Can you work these out from the model? Positions are in its coordinate system, mm. Face numbers are marked on the shaded views. A direction names the side the tool comes from. Round coordinates to 2 decimals unless told otherwise and drop trailing zeros. Loops run counter-clockwise (first coordinate to the right, second up) from the corner with the lowest first, then second, coordinate; pieces in that order, holes last. Notation, with made-up numbers: (66, 11.25) -> (77, 11.25) arc R19 ccw to (77, 27.25) -> close; hole circle Ø1 at (-7.75, -39). An arc over 180 degrees is marked (long way). Use a Markdown table: item, result.
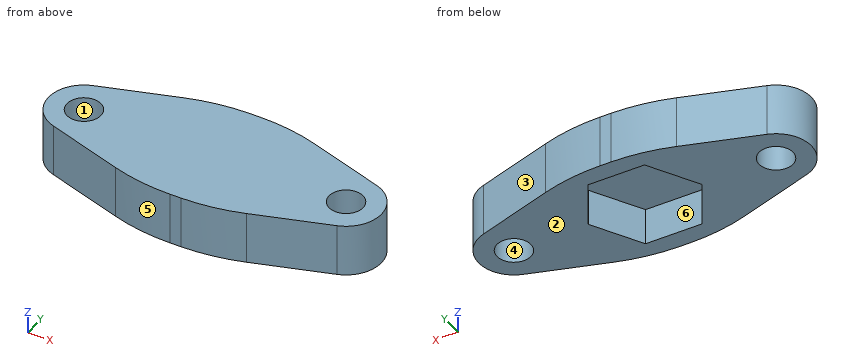
from build123d import *

# Parameters (mm, degrees)
SKETCH1_R           = 1.3
BOSS_EXTRUDE1_DEPTH = 4
SKETCH2_R           = 4.330127019
BOSS_EXTRUDE2_DEPTH = 1.2


with BuildPart() as part:
    # Sketch1 → Boss-Extrude1 (new body)
    with BuildSketch(Plane.XY):
        with BuildLine():
            Line((10.823243212, 2.571433572), (5, 4.435742065))
            ThreePointArc((5, 4.435742065), (2.74093184, 4.97035983), (0.426426599, 5.15))
            Line((0.426426599, 5.15), (-0.426426599, 5.15))
            ThreePointArc((-0.426426599, 5.15), (-2.74093184, 4.97035983), (-5, 4.435742065))
            Line((-5, 4.435742065), (-10.823243212, 2.571433572))
            ThreePointArc((-10.823243212, 2.571433572), (-12.7, 0), (-10.823243212, -2.571433572))
            Line((-10.823243212, -2.571433572), (-5, -4.435742065))
            ThreePointArc((-5, -4.435742065), (-2.74093184, -4.97035983), (-0.426426599, -5.15))
            Line((-0.426426599, -5.15), (0.426426599, -5.15))
            ThreePointArc((0.426426599, -5.15), (2.74093184, -4.97035983), (5, -4.435742065))
            Line((5, -4.435742065), (10.823243212, -2.571433572))
            ThreePointArc((10.823243212, -2.571433572), (12.7, 0), (10.823243212, 2.571433572))
        make_face()
        with Locations((10, 0)):
            Circle(SKETCH1_R, mode=Mode.SUBTRACT)
        with Locations(Location((-10, 0, 0), (0, 0, 180))):
            Circle(SKETCH1_R, mode=Mode.SUBTRACT)
        Polygon((2.165063509, 3.75), (-2.165063509, 3.75), (-4.330127019, 0), (-2.165063509, -3.75), (2.165063509, -3.75), (4.330127019, 0), align=None, mode=Mode.SUBTRACT)
    extrude(amount=BOSS_EXTRUDE1_DEPTH)

    # Sketch2 → Boss-Extrude2 (add)
    with BuildSketch(Plane.XY.offset(4)):
        Circle(SKETCH2_R)
    extrude(amount=-BOSS_EXTRUDE2_DEPTH)


solid = part.part
1. I want a section at B-B (y = -0.5). Please give me the cut outline in (x, z), plus the area to 3 significant figures.
Answer sheet:
| item | result |
|---|---|
| outline | (-12.65, 0) -> (-11.2, 0) -> (-11.2, 4) -> (-12.65, 4) -> close; (-8.8, 0) -> (-4.04, 0) -> (-4.04, 2.8) -> (4.04, 2.8) -> (4.04, 0) -> (8.8, 0) -> (8.8, 4) -> (-8.8, 4) -> close; (11.2, 0) -> (12.65, 0) -> (12.65, 4) -> (11.2, 4) -> close |
| area | 59.4 mm² |
2. Will these pins go through, and if not, where does the flat tip stop? pin 1 Ø1 at (x, z) = (-3, 1.5) entering from +Y; pin 2 Ø1.6 at (x, y) = (10, 0) entering from -Z.
Answer sheet:
| item | result |
|---|---|
| pin 1 | stops at y = 5.01 |
| pin 2 | passes through |
3. I need wall thicknesses on line 1 (Z direction, x = 1, y = -1.75); line 2 (Y direction, x = -10, z = 2.5) (3 decimals); line 3 (X direction, y = 0.5, z = 3.15). Which ranges of each line are inside material? Lowest first, please.
Answer sheet:
| item | result |
|---|---|
| line 1 | z = 2.8 to 4 |
| line 2 | y = -2.835 to -1.3, 1.3 to 2.835 |
| line 3 | x = -12.65 to -11.2, -8.8 to 8.8, 11.2 to 12.65 |
4. If we mould it in two halves opening along Y, with no side actions, what happens to the marked faces 1, 2, 3 and 4? For each: +Y half, -Y half, draft (parallel to the pull), parting line (faces both ways), or undercut.
Answer sheet:
| item | result |
|---|---|
| face 1 | undercut |
| face 2 | draft |
| face 3 | +Y half |
| face 4 | undercut |
5. Which directions (+Z, -Z, +X, -X, +Y, -Y) give clear straight access to the entire face, cutting with the end or side of a thin tool? Please do the marked faces 5 and 6.
Answer sheet:
| item | result |
|---|---|
| face 5 | +Z, -Z, -X, -Y |
| face 6 | -Z |
6. I want a section at A-A (z = 2.35). Please give me the cut outline in (x, y).
Answer sheet:
| item | result |
|---|---|
| outline | (-10.82, -2.57) -> (-5, -4.44) arc R15 ccw to (-0.43, -5.15) -> (0.43, -5.15) arc R15 ccw to (5, -4.44) -> (10.82, -2.57) arc R2.7 ccw to (10.82, 2.57) -> (5, 4.44) arc R15 ccw to (0.43, 5.15) -> (-0.43, 5.15) arc R15 ccw to (-5, 4.44) -> (-10.82, 2.57) arc R2.7 ccw to start; hole circle Ø2.6 at (-10, 0); hole (-4.33, 0) -> (-2.17, -3.75) -> (2.17, -3.75) -> (4.33, 0) -> (2.17, 3.75) -> (-2.17, 3.75) -> close; hole circle Ø2.6 at (10, 0) |
7. I want a section at D-D (y = -2.25). Please give me the cut outline in (x, z), plus the area to 3 significant figures.
Answer sheet:
| item | result |
|---|---|
| outline | (-11.49, 0) -> (-3.03, 0) -> (-3.03, 2.8) -> (3.03, 2.8) -> (3.03, 0) -> (11.49, 0) -> (11.49, 4) -> (-11.49, 4) -> close |
| area | 75.0 mm² |
8. I want a section at C-C (x = -10). Please give me the cut outline in (y, z) (3 decimals).
Answer sheet:
| item | result |
|---|---|
| outline | (-2.835, 0) -> (-1.3, 0) -> (-1.3, 4) -> (-2.835, 4) -> close; (1.3, 0) -> (2.835, 0) -> (2.835, 4) -> (1.3, 4) -> close |
